```python
from build123d import *

# Parameters (mm, degrees)
ESQUISSE1_W      = 25
ESQUISSE1_H      = 25
ESQUISSE1_R      = 1.5
ESQUISSE1_R_2    = 3
EXTRUSION3_DEPTH = 30
ESQUISSE8_R      = 10
EXTRUSION4_DEPTH = 28
ESQUISSE10_R     = 18.049415766
ESQUISSE10_R_2   = 12.5
EXTRUSION6_DEPTH = 2


with BuildPart() as part:
    # Esquisse1 → Extrusion3 (new body)
    with BuildSketch(Plane.XY):
        Rectangle(ESQUISSE1_W, ESQUISSE1_H)
        with Locations((10, 10)):
            Circle(ESQUISSE1_R, mode=Mode.SUBTRACT)
        Circle(ESQUISSE1_R_2, mode=Mode.SUBTRACT)
        with Locations((-10, 10)):
            Circle(ESQUISSE1_R, mode=Mode.SUBTRACT)
        with Locations((10, -10)):
            Circle(ESQUISSE1_R, mode=Mode.SUBTRACT)
        with Locations((-10, -10)):
            Circle(ESQUISSE1_R, mode=Mode.SUBTRACT)
    extrude(amount=EXTRUSION3_DEPTH)

    # Esquisse8 → Extrusion4 (cut)
    with BuildSketch(Plane.XY.offset(30)):
        Circle(ESQUISSE8_R)
    extrude(amount=-EXTRUSION4_DEPTH, mode=Mode.SUBTRACT)

    # Esquisse10 → Extrusion6 (cut)
    with BuildSketch(Plane.XY.offset(30)):
        Circle(ESQUISSE10_R)
        Circle(ESQUISSE10_R_2, mode=Mode.SUBTRACT)
    extrude(amount=-EXTRUSION6_DEPTH, mode=Mode.SUBTRACT)


solid = part.part
```
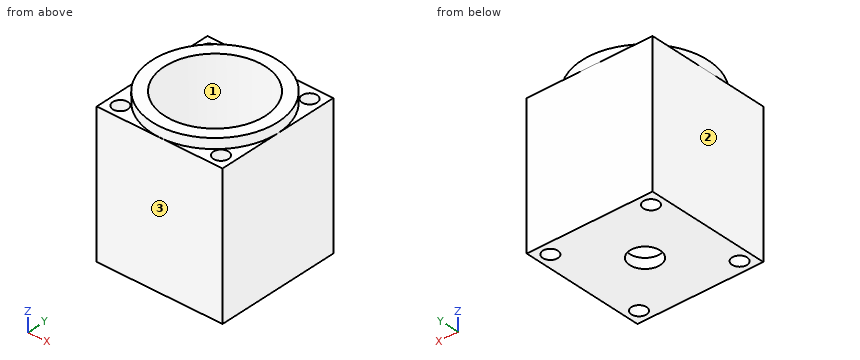
Part model, mm, in its own coordinate system. Face numbers are marked on the shaded views. Give positions to 0.01 mm unless a question says otherwise; leave off trailing zeros. Write each loop counter-clockwise with the first axis right and the second up, starting at its lowest first coordinate (ties: lowest second). Pieces come first, ordered by that corner, then holes. Notation, with made-up numbers: (73, 29) -> (132, 29) arc R13 cw to (132, 39) -> close; hole circle Ø3 at (3, 47.25). An arc over 180 degrees is marked (long way). Put each result on its own line as item: value. Start each with the question number.
Item 1: Cut at C-C (x = -10.5). List the corners of the cut face in (y, z), then the cut area to 3 significant figures.
Item 2: Wall check: L1, parallel to Y at x = 0, z = 0.95; L2, parallel to X at y = 8.75, z = 22.75; L3, parallel to Y at x = 9, z = 6. Give the ranges that are in metal, low to high. Write a range as [from, to].
Item 3: Cut at A-A (z = 8.25). List the corners of the cut face in (x, y), then the cut area to 3 significant figures.
Item 4: Cut at B-B (y = 1.25). List the corners of the cut face in (x, z).
Item 5: Pin check, flat tips, straight feed: pin 1 Ø14 at (x, y) = (-6.5, 6) entering from +Z; pin 2 Ø9.5 at (x, y) = (0, 0) entering from +Z. Stop position of each tip, or through.
Item 6: Pull direction X, two halves, no side cores. Call the marked faces 1, 2 and 3: pulls with the +X half, pulls with the -X half, needs draft (parallel to the pull), parting line crosses it, or undercut.
Answer list:
1. outline: (-12.5, 0) -> (-11.41, 0) -> (-11.41, 28) -> (-12.5, 28) -> close; (-8.59, 0) -> (8.59, 0) -> (8.59, 28) -> (6.78, 28) -> (6.78, 30) -> (-6.78, 30) -> (-6.78, 28) -> (-8.59, 28) -> close; (11.41, 0) -> (12.5, 0) -> (12.5, 28) -> (11.41, 28) -> close
1. area: 569 mm2
2. L1: y = [-12.5, -3], [3, 12.5]
2. L2: x = [-12.5, -10.83], [-9.17, -4.84], [4.84, 9.17], [10.83, 12.5]
2. L3: y = [-12.5, -11.12], [-8.88, -4.36], [4.36, 8.88], [11.12, 12.5]
3. outline: (-12.5, -12.5) -> (12.5, -12.5) -> (12.5, 12.5) -> (-12.5, 12.5) -> close; hole circle Ø3 at (-10, -10); hole circle Ø3 at (-10, 10); hole circle Ø20 at (0, 0); hole circle Ø3 at (10, -10); hole circle Ø3 at (10, 10)
3. area: 283 mm2
4. outline: (-12.5, 0) -> (-2.73, 0) -> (-2.73, 2) -> (-9.92, 2) -> (-9.92, 30) -> (-12.44, 30) -> (-12.44, 28) -> (-12.5, 28) -> close; (2.73, 0) -> (12.5, 0) -> (12.5, 28) -> (12.44, 28) -> (12.44, 30) -> (9.92, 30) -> (9.92, 2) -> (2.73, 2) -> close
5. pin 1: stops at z = 30
5. pin 2: stops at z = 2
6. face 1: undercut
6. face 2: pulls with the -X half
6. face 3: needs draft
